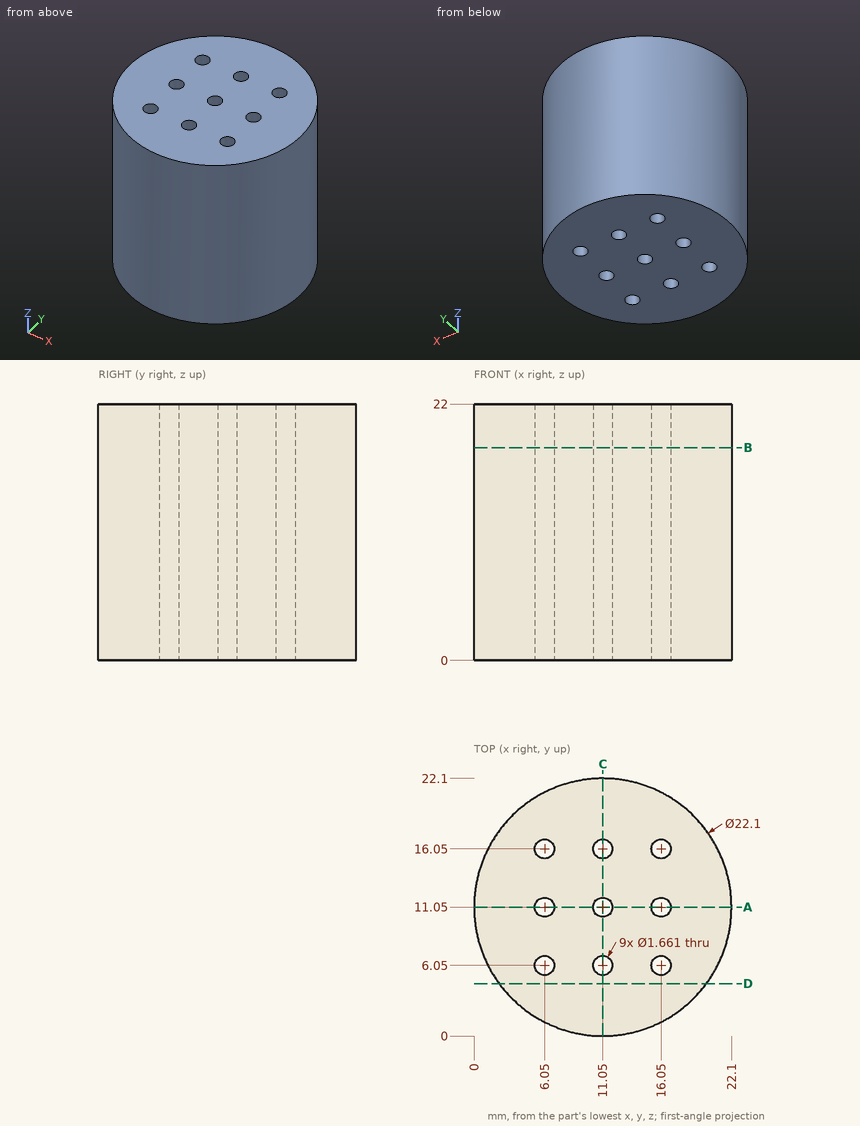
Verification items for this drawing (mm, ordinates from the low corner). Round coordinates to 2 decimals unless told otherwise and drop trailing zeros. Loops run counter-clockwise (first coordinate to the right, second up) from the corner with the lowest first, then second, coordinate; pieces in that order, holes last. Notation, with made-up numbers: (-4.75, 34) -> (35.25, 34) arc R22 cw to (35.25, 71) -> close; hole circle Ø9 at (33, -19.5). An arc over 180 degrees is marked (long way). Write item = value, one per line. Start each with the question number.
1) Sectioned sample at B-B, the plane z = 18.25. State how many separate pieces and enclosed holes the cut face has, plus the area to 3 significant figures.
2) Gauge pin test, flat ends, axial feed: pin 1 Ø5 at (x, z) = (2.5, 4) entering from -Y; pin 2 Ø5 at (y, z) = (19, 8) entering from +X. Record the tip position at first contact, or that the pin passes through.
3) Thickness scan on probe 1 along X at (y, z) = (16.75, 18.25) (1 decimal); probe 2 along Y at (x, z) = (16.05, 9); probe 3 along X at (y, z) = (16, 21). Record the ranges inside material, lowest first.
4) Sectioned sample at D-D, the plane y = 4.5. Record the cut outline in (x, z), plus the area to 3 significant figures.
5) Sectioned sample at A-A, the plane y = 11.05. Record the cut outline in (x, z).
Results are:
q1.separate_pieces = 1
q1.enclosed_holes = 9
q1.area = 364 mm^2
q2.pin_1 = 1.8
q2.pin_2 = 20.66
q3.probe_1 = 1.6 to 5.6, 6.5 to 10.6, 11.5 to 15.6, 16.5 to 20.5
q3.probe_2 = 1.2 to 5.22, 6.88 to 10.22, 11.88 to 15.22, 16.88 to 20.9
q3.probe_3 = 1.17 to 5.22, 6.88 to 10.22, 11.88 to 15.22, 16.88 to 20.93
q4.outline = (2.15, 0) -> (19.95, 0) -> (19.95, 22) -> (2.15, 22) -> close
q4.area = 392 mm^2
q5.outline = (0, 0) -> (5.22, 0) -> (5.22, 22) -> (0, 22) -> close; (6.88, 0) -> (10.22, 0) -> (10.22, 22) -> (6.88, 22) -> close; (11.88, 0) -> (15.22, 0) -> (15.22, 22) -> (11.88, 22) -> close; (16.88, 0) -> (22.1, 0) -> (22.1, 22) -> (16.88, 22) -> close
